Source: CAD feature listing. Evaluate the final solid. Frame: model axes, mm. A direction names the side the tool comes from. Coordinates: 2 decimals unless noted, no trailing zeros. Write each loop counter-clockwise with the first axis right and the second up, starting at its lowest first coordinate (ties: lowest second). Pieces come first, ordered by that corner, then holes. Notation, with made-up numbers: M -4,68.25 L 13,68.25 A21 ccw 13,72.25 Z; hole C -17,17 d6. An arc over 180 degrees is marked long. One line per item, written item: value. Start each with the question number.
Item 1: Ray query, L1, parallel to Y at x = 7, z = 2.25; L2, parallel to Z at x = 0, y = 2.25; L3, parallel to Z at x = -7.75, y = 9.25. Return the intervals inside material, ascending. Write a range as from..to.
Item 2: Cut plane A-A, the plane x = 5. Output: boundary loops of the cut face in (y, z), then the cut area to 3 significant figures.
Item 3: Cut plane D-D, the plane x = -4.5. Output: boundary loops of the cut face in (y, z), then the cut area to 3 significant figures.
Item 4: Pin query (flat end, axial travel): P1, Ø0.6, axis at y = -0.5, z = 0.5, coming from the -X side; P2, Ø4, axis at y = 4, z = -2, coming from the -X side. Return the tip coordinate at first contact, or that it passes through.
Item 5: Cut plane B-B, the plane z = 6. Output: boundary loops of the cut face in (x, y).
Item 6: Cut plane C-C, the plane y = 3.5. Output: boundary loops of the cut face in (x, z).
Item 7: Mould query, pull axis Y, two halves, no side actions, for faces 1 (the flat face through (-2, 0, 0)), 2 (the flat face through (-1, 4, -7.4)), 3 (the flat face through (3, 9.5, -3)). Classes: released by +Y, released by -Y, zero draft, split by the parting line, or undercut.
Item 8: Set-up query: faces 4 (the flat face through (-8.3, -1, 0)), 5 (the flat face through (-5, 8, 4)), 6 (the flat face through (-1, 4, -6.6)), 7 (the flat face through (-9, 1.4, 7)), 8 (the flat face through (-10.3, 8, -6)). Return all of +Z, -Z, +X, -X, +Y, -Y with unobstructed straight access to the full face (end or side cutting, diameter ignored); none if empty.
```python
from build123d import *

# Parameters (mm, degrees)
BOSS_EXTRUDE1_DEPTH = 7.5
SKETCH4_W           = 16.6
SKETCH4_H           = 14.8
BOSS_EXTRUDE2_DEPTH = 2
BOSS_EXTRUDE3_DEPTH = 2
BOSS_EXTRUDE6_DEPTH = 2


with BuildPart() as part:
    # Sketch3 → Boss-Extrude1 (new body)
    with BuildSketch(Plane(origin=(0, 0, 0), x_dir=(1, 0, 0), z_dir=(0, 1, 0))):
        Polygon((8.3, -7.4), (8.3, 7.4), (-8.3, 7.4), (-8.3, 6.6), (-7.5, 6.6), (7.5, 6.6), (7.5, -6.6), (-7.5, -6.6), (-8.3, -6.6), (-8.3, -7.4), align=None)
    extrude(amount=BOSS_EXTRUDE1_DEPTH)

    # Sketch4 → Boss-Extrude2 (add)
    with BuildSketch(Plane.XZ):
        Rectangle(SKETCH4_W, SKETCH4_H)
    extrude(amount=BOSS_EXTRUDE2_DEPTH)

    # Sketch5 → Boss-Extrude3 (add)
    with BuildSketch(Plane(origin=(0, 7.5, 0), x_dir=(1, 0, 0), z_dir=(0, 1, 0))):
        with BuildLine():
            Line((-8.3, 4), (0, 4))
            ThreePointArc((0, 4), (4, 0), (0, -4))
            Line((0, -4), (-8.3, -4))
            Line((-8.3, -4), (-8.3, -7.4))
            Line((-8.3, -7.4), (8.3, -7.4))
            Line((8.3, -7.4), (8.3, 7.4))
            Line((8.3, 7.4), (-8.3, 7.4))
            Line((-8.3, 7.4), (-8.3, 4))
        make_face()
    extrude(amount=BOSS_EXTRUDE3_DEPTH)

    # Sketch8 → Boss-Extrude6 (add)
    with BuildSketch(Plane.ZY.offset(8.3)):
        Polygon((-4, 9.5), (-7.4, 9.5), (-7.4, 6.1), (-6.6, 6.1), (-6.6, 7.5), (-4, 7.5), align=None)
        Polygon((4, 9.5), (4, 7.5), (6.6, 7.5), (6.6, 6.1), (7.4, 6.1), (7.4, 9.5), align=None)
        Polygon((6.6, 1.4), (7.4, 1.4), (7.4, -2), (4, -2), (4, 0), (6.6, 0), align=None)
        Polygon((-7.4, 1.4), (-6.6, 1.4), (-6.6, 0), (-4, 0), (-4, -2), (-7.4, -2), align=None)
    extrude(amount=BOSS_EXTRUDE6_DEPTH)


solid = part.part
```
From the geometry:
1. L1: y = -2..0, 7.5..9.5
1. L2: z = -7.4..-6.6, 6.6..7.4
1. L3: z = -7.4..-4, 4..7.4
2. outline: M -2,-7.4 L 9.5,-7.4 L 9.5,7.4 L -2,7.4 Z; hole M 0,-6.6 L 7.5,-6.6 L 7.5,6.6 L 0,6.6 Z
2. area: 71.2 mm²
3. outline: M -2,-7.4 L 9.5,-7.4 L 9.5,-4 L 7.5,-4 L 7.5,-6.6 L 0,-6.6 L 0,6.6 L 7.5,6.6 L 7.5,4 L 9.5,4 L 9.5,7.4 L -2,7.4 Z
3. area: 55.2 mm²
4. P1: stops at x = -8.3
4. P2: stops at x = 7.5
5. outline: M -10.3,-2 L 8.3,-2 L 8.3,9.5 L -10.3,9.5 L -10.3,7.5 L 7.5,7.5 L 7.5,0 L -10.3,0 Z
6. outline: M -8.3,-7.4 L 8.3,-7.4 L 8.3,7.4 L -8.3,7.4 L -8.3,6.6 L 7.5,6.6 L 7.5,-6.6 L -8.3,-6.6 Z
7. face 1: undercut
7. face 2: zero draft
7. face 3: released by +Y
8. face 4: -X, +Y, -Y
8. face 5: -X, +Y
8. face 6: -X
8. face 7: +Z, -Z, -X
8. face 8: +Z, -Z, -X, +Y, -Y
